Part model, mm, in its own coordinate system. Face numbers are marked on the shaded views. A direction names the side the tool comes from. Coordinates: 2 decimals unless noted, no trailing zeros. Loops run counter-clockwise (first coordinate to the right, second up) from the corner with the lowest first, then second, coordinate; pieces in that order, holes last. Notation, with made-up numbers: (64, 85) -> (120, 85) arc R28 cw to (120, 121) -> close; hole circle Ø7 at (43.5, 36). An arc over 180 degrees is marked (long way). One line per question, with ' | ' between items. Start each with the question number.
1) Probe L1, parallel to X at y = -1.6, z = 1.65; L2, parallel to Z at x = 1.5, y = 0.05; L3, parallel to Z at x = 8.5, y = -0.4. List the from-to ranges inside material, lowest first. Write a range as from..to.
2) Two-plate mould, pull along Z, no slides. Class the marked faces 1, 2, 3 and 4: released by +Z, released by -Z, zero draft, split by the parting line, or undercut.
3) Cut at A-A (x = 5.75). List the corners of the cut face in (y, z), plus the area to 3 significant figures.
4) 3-axis set-ups, long thin cutter, end or side, ignore diameter. For the marked faces 5, 6 and 7: which of +Z, -Z, +X, -X, +Y, -Y reach the whole face in a straight line?
5) Drop a flat-ended pin along its axis: pin 1 (3 mm diameter, centred on x = 7, y = 1, fed in from -Z). Give the stop position or say it passes through.
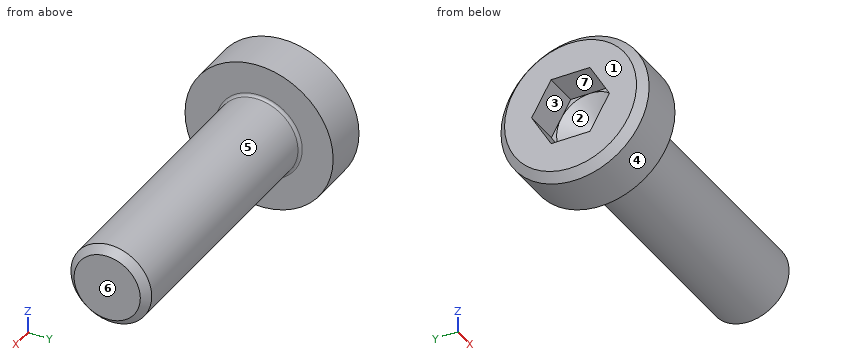
Autodesk Inventor part; units mm, degrees
ref_plane "SCW_XY" through (0, 0, 0) normal (1, 0, 0) x (0, 0, -1)
ref_plane "SCW_YZ" through (0, 0, 0) normal (0, 0, -1) x (0, 1, 0)
ref_plane "SCW_ZX" through (0, 0, 0) normal (0, 1, 0) x (1, 0, 0)
sketch "Sketch_1" plane through (0, 0, 0) normal (0, 0, 1) x (1, 0, 0)
  line L0 (10, 0) -> (-2, 0)
  line L1 (-2, 0) -> (-2, 2.45)
  line L2 (-2, 2.45) -> (-1.7, 2.75)
  line L3 (-1.7, 2.75) -> (0, 2.75)
  line L4 (0, 2.75) -> (0, 1.6)
  arc A0 (0, 1.6) -> (0.1, 1.5) centre (0.1, 1.6) ccw
  line L5 (0.1, 1.5) -> (9.7295, 1.5)
  line L6 (9.7295, 1.5) -> (10, 1.2295)
  line L7 (10, 1.2295) -> (10, 0)
  line L8 (10, 0) -> (-2, 0)
revolve "Revolution1" add sketch "Sketch_1" angle 360 about axis through (10, 0, 0) along (1, 0, 0)
thread "Thread1"
sketch "Sketch_2" plane through (-2, 0, 0) normal (1, 0, 0) x (0, 0, -1)
  line L0 (-1.25, 0.7217) -> (-1.25, -0.7217)
  line L1 (-1.25, -0.7217) -> (0, -1.4434)
  line L2 (0, -1.4434) -> (1.25, -0.7217)
  line L3 (1.25, -0.7217) -> (1.25, 0.7217)
  line L4 (1.25, 0.7217) -> (0, 1.4434)
  line L5 (0, 1.4434) -> (-1.25, 0.7217)
extrude "Extrusion1" cut sketch "Sketch_2" along normal blind 1.3
sketch "Sketch_5" plane through (0, 0, 0) normal (0, 0, 1) x (1, 0, 0)
  line L0 (0.0217, 0) -> (-0.7, 0)
  line L1 (-0.7, 0) -> (-0.7, 1.25)
  line L2 (-0.7, 1.25) -> (0.0217, 0)
  line L3 (0.0217, 0) -> (-0.7, 0)
revolve "Revolution2" cut sketch "Sketch_5" angle 360 about axis through (0.0217, 0, 0) along (1, 0, 0)
ref_plane "SCW_XY" through (0, 0, 0) normal (1, 0, 0) x (0, 0, -1)
ref_plane "SCW_YZ" through (0, 0, 0) normal (0, 0, -1) x (0, 1, 0)
ref_plane "SCW_ZX" through (0, 0, 0) normal (0, 1, 0) x (1, 0, 0)
properties part number "M3-10_bo"
Reported:
1) L1: x = -2..0 | L2: z = -1.5..1.5 | L3: z = -1.45..1.45
2) face 1: zero draft | face 2: undercut | face 3: undercut | face 4: split by the parting line
3) outline: circle Ø3 at (0, 0) | area: 7.07 mm²
4) face 5: +X | face 6: +Z, -Z, +X, +Y, -Y | face 7: -X
5) pin 1: stops at z = -1.5
